```python
from build123d import *

# Parameters (mm, degrees)
ESBO_O1_W                = 167
ESBO_O1_H                = 50
RESSALTO_EXTRUS_O1_DEPTH = 6
ESBO_O3_R                = 3
CORTE_EXTRUS_O1_DEPTH    = 20


with BuildPart() as part:
    # Esboço1 → Ressalto-extrusão1 (new, symmetric)
    with BuildSketch(Plane.XY):
        Rectangle(ESBO_O1_W, ESBO_O1_H)
    extrude(amount=RESSALTO_EXTRUS_O1_DEPTH, both=True)

    # Esboço3 → Corte-extrusão1 (cut)
    with BuildSketch(Plane(origin=(0, -25, 0), x_dir=(-1, 0, 0), z_dir=(0, -1, 0))):
        with Locations(Location((75, 0, 0), (0, 0, 90))):
            Circle(ESBO_O3_R)
        with Locations(Location((-75, 0, 0), (0, 0, 90))):
            Circle(ESBO_O3_R)
    extrude(amount=-CORTE_EXTRUS_O1_DEPTH, mode=Mode.SUBTRACT)


solid = part.part
```
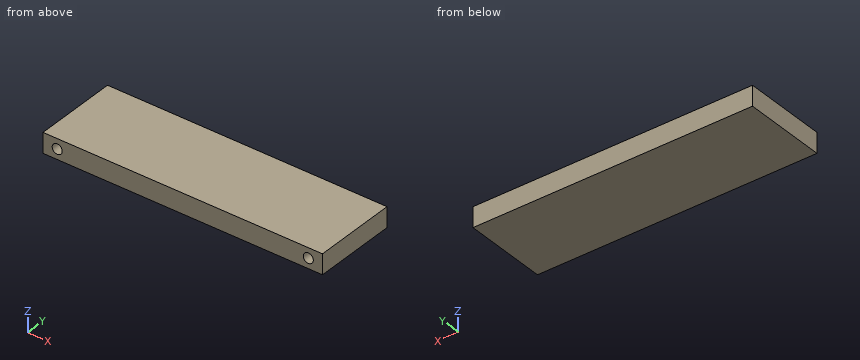
For this review, take the finished solid that the model builds, in its own axes (mm). Round coordinates to 2 decimals unless told otherwise and drop trailing zeros. Write each loop counter-clockwise with the first axis right and the second up, starting at its lowest first coordinate (ties: lowest second). Pieces come first, ordered by that corner, then holes. Notation, with made-up numbers: M -28.75,-17 L -9.75,-17 A29 cw -9.75,4 Z; hole C -21,31 d3. An arc over 180 degrees is marked long. One line per item, written item: value. Start each with the question number.
(1) We need section C-C (y = -14). Give the boundary of the cut face in (x, z).
(2) Insertion check: pin 1 (3.5 mm diameter, centred on x = 75, z = 0, fed in from -Y). The pin has a flat end and moves straight along its axis. Give the tip position at first contact, or say it passes through.
(3) We need section B-B (x = -75). Give the boundary of the cut face in (y, z), and give its area (3 significant figures).
(4) Wall thickness on line 1 (X direction, y = -10.5, z = 0); line 2 (X direction, y = -14.5, z = 1.75): over which ranges is each line inside the solid? List them lowest first.
(5) We need section A-A (z = 0). Give the boundary of the cut face in (x, y), and give its area (3 significant figures).
Result:
1. outline: M -83.5,-6 L 83.5,-6 L 83.5,6 L -83.5,6 Z; hole C -75,0 d6; hole C 75,0 d6
2. pin 1: y = -5
3. outline: M -25,-6 L 25,-6 L 25,6 L -25,6 L -25,3 L -5,3 L -5,-3 L -25,-3 Z
3. area: 480 mm²
4. line 1: -83.5 to -78, -72 to 72, 78 to 83.5
4. line 2: -83.5 to -77.44, -72.56 to 72.56, 77.44 to 83.5
5. outline: M -83.5,-25 L -78,-25 L -78,-5 L -72,-5 L -72,-25 L 72,-25 L 72,-5 L 78,-5 L 78,-25 L 83.5,-25 L 83.5,25 L -83.5,25 Z
5. area: 8,110 mm²
